from build123d import *

# Parameters (mm, degrees)
BOSS_EXTRUDE1_DEPTH = 2.54


with BuildPart() as part:
    # Sketch1 → Boss-Extrude1 (new body)
    with BuildSketch(Plane.XY):
        with BuildLine():
            ThreePointArc((-13.324567367, -3.22122711), (-9.201637253, 5.466316018), (0, 2.673140373))
            ThreePointArc((0, 2.673140373), (9.201637253, 5.466316018), (13.324567367, -3.22122711))
            ThreePointArc((13.324567367, -3.22122711), (10.447333261, -9.42774786), (5.704348435, -14.357602914))
            ThreePointArc((5.704348435, -14.357602914), (2.946415451, -16.171190718), (0, -17.659119163))
            ThreePointArc((0, -17.659119163), (-2.946415451, -16.171190718), (-5.704348435, -14.357602914))
            ThreePointArc((-5.704348435, -14.357602914), (-10.447333261, -9.42774786), (-13.324567367, -3.22122711))
        make_face()
        with BuildLine():
            ThreePointArc((12.344862067, -2.952092336), (7.698572292, 4.905869161), (0, 0))
            ThreePointArc((0, 0), (-7.698572292, 4.905869161), (-12.344862067, -2.952092336))
            ThreePointArc((-12.344862067, -2.952092336), (-9.608841906, -8.853998571), (-5.098641611, -13.541897549))
            ThreePointArc((-5.098641611, -13.541897549), (-2.629119582, -15.179915612), (0, -16.547165572))
            ThreePointArc((0, -16.547165572), (2.629119582, -15.179915612), (5.098641611, -13.541897549))
            ThreePointArc((5.098641611, -13.541897549), (9.608841906, -8.853998571), (12.344862067, -2.952092336))
        make_face(mode=Mode.SUBTRACT)
    extrude(amount=BOSS_EXTRUDE1_DEPTH)


solid = part.part
Input: part model. Units: mm. Frame: model coordinates. A direction names the side the tool comes from. Coordinates: 2 decimals unless noted, no trailing zeros. Loops run counter-clockwise (first coordinate to the right, second up) from the corner with the lowest first, then second, coordinate; pieces in that order, holes last. Notation, with made-up numbers: (75.5, 86.25) -> (106.5, 86.25) arc R29 cw to (106.5, 123.25) -> close; hole circle Ø2 at (89.25, -32.5). An arc over 180 degrees is marked (long way). Write item = value, one per line. Start each with the question number.
Item 1: Cut plane A-A, the plane y = -1.27. Return loops of the section in (x, z).
Item 2: Reachability of faces 4 (the face through (0, 1, 2.54)), 5 (the face through (9.557, -8.929, 1.252)) from +Z, -Z, +X, -X, +Y, -Y: full face, straight path, thin tool, end or side. Return the list, or none.
Item 3: Cut plane D-D, the plane y = -11.75. Return loops of the section in (x, z), plus the area to 3 significant figures.
Item 4: Material intervals for line 1 (X direction, y = 3.5, z = 2.4); line 2 (X direction, y = -4.25, z = 1.05); line 3 (X direction, y = -1.75, z = 1.4), sorted ascending.
Item 5: Cut plane B-B, the plane y = 2.25. Return loops of the section in (x, z).
Item 6: Mould query, pull axis X, two halves, no side actions, for faces 1 (the face through (7.84, 4.87, 1.25)), 2 (the face through (10.5, -9.35, 1.25)), 3 (the face through (0, 1, 0)). Classes: pulls with the +X half, pulls with the -X half, needs draft (parallel to the pull), parting line crosses it, or undercut.
Item 7: First-contact query: P1, Ø1, axis at x = -1.5, z = 2, coming from the +Y side; P2, Ø1, axis at x = 10.5, z = 2, coming from the +Y side; P3, Ø1, axis at y = 0, z = 1, coming from the -X side. Flat tips, straight axial feed; report the tip coordinate or a pass-through.
Item 8: Cut plane C-C, the plane z = 1.2. Return loops of the section in (x, y) (3 decimals).
Ans:
q1.outline = (-13.59, 0) -> (-12.57, 0) -> (-12.57, 2.54) -> (-13.59, 2.54) -> close; (12.57, 0) -> (13.59, 0) -> (13.59, 2.54) -> (12.57, 2.54) -> close
q2.face_4 = +Z, +X, -X, +Y, -Y
q2.face_5 = +Z, -Z
q3.outline = (-8.6, 0) -> (-7.19, 0) -> (-7.19, 2.54) -> (-8.6, 2.54) -> close; (7.19, 0) -> (8.6, 0) -> (8.6, 2.54) -> (7.19, 2.54) -> close
q3.area = 7.17 mm²
q4.line_1 = -11.83 to -10.41, -2.03 to -0.61, 0.61 to 2.03, 10.41 to 11.83
q4.line_2 = -13.01 to -11.94, 11.94 to 13.01
q4.line_3 = -13.57 to -12.55, 12.55 to 13.57
q5.outline = (-12.69, 0) -> (-11.51, 0) -> (-11.51, 2.54) -> (-12.69, 2.54) -> close; (-0.94, 0) -> (0.94, 0) -> (0.94, 2.54) -> (-0.94, 2.54) -> close; (11.51, 0) -> (12.69, 0) -> (12.69, 2.54) -> (11.51, 2.54) -> close
q6.face_1 = undercut
q6.face_2 = pulls with the +X half
q6.face_3 = needs draft
q7.P1 = 4.77
q7.P2 = 5.05
q7.P3 = -13.55
q8.outline = (-13.325, -3.221) arc R20.701 ccw to (-5.704, -14.358) arc R28.956 ccw to (0, -17.659) arc R28.956 ccw to (5.704, -14.358) arc R20.701 ccw to (13.325, -3.221) arc R7.366 ccw to (0, 2.673) arc R7.366 ccw to start; hole (-12.345, -2.952) arc R19.685 ccw to (-5.099, -13.542) arc R27.94 ccw to (0, -16.547) arc R27.94 ccw to (5.099, -13.542) arc R19.685 ccw to (12.345, -2.952) arc R6.35 ccw (long way) to (0, 0) arc R6.35 ccw (long way) to start
